from build123d import *
from build123d.topology import SkipClean

# Parameters (mm, degrees)
SKETCH1_W               = 29.21
SKETCH1_H               = 55.1434
BOSS_EXTRUDE1_DEPTH     = 55.88
SKETCH2_R               = 12.065
CUT_REVOLVE1_ANGLE      = 90
SKETCH3_R               = 25.4
CUT_EXTRUDE1_DEPTH      = 43.18
CUT_EXTRUDE4_DEPTH      = 2.0955
CUT_EXTRUDE4_DEPTH_BACK = 0.508
SKETCH6_R               = 23.8125
SKETCH7_R               = 2.6543
CUT_EXTRUDE5_DEPTH      = 7.62
CHAMFER1_SIZE           = 7.62
CHAMFER1_SIZE2          = 13.198227154
SKETCH8_R               = 2.6543
CUT_EXTRUDE6_DEPTH      = 7.62
SKETCH9_R               = 2.6543
CUT_EXTRUDE7_DEPTH      = 7.62


with BuildPart() as part:
    # Sketch1 → Boss-Extrude1 (new body)
    with BuildSketch(Plane(origin=(0, 0, 0), x_dir=(1, 0, 0), z_dir=(0, 1, 0))):
        with Locations((0, -27.5717)):
            Rectangle(SKETCH1_W, SKETCH1_H)
    extrude(amount=BOSS_EXTRUDE1_DEPTH)

    # Sketch2 → Cut-Revolve1 (revolve, cut)
    with BuildSketch(Plane(origin=(0, 0, 0), x_dir=(-1, 0, 0), z_dir=(0, 0, -1))):
        with Locations((0, 40.5384)):
            Circle(SKETCH2_R)
    revolve(axis=Axis((14.605, 0, 0), (1, 0, 0)), revolution_arc=CUT_REVOLVE1_ANGLE, mode=Mode.SUBTRACT)

    # Sketch3 → Cut-Extrude1 (cut)
    with BuildSketch(Plane(origin=(0, 55.88, 0), x_dir=(1, 0, 0), z_dir=(0, 1, 0))):
        with Locations((-29.0576, 0)):
            Circle(SKETCH3_R)
        with Locations((29.0576, 0)):
            Circle(SKETCH3_R)
    extrude(amount=-CUT_EXTRUDE1_DEPTH, mode=Mode.SUBTRACT)

    # Sketch6 → Cut-Extrude4 (cut, two sides: drawn at the far end of the back side and taken through both)
    with SkipClean():  # the faces are left unmerged after this step: merging them gives an invalid solid
        with BuildSketch(Plane(origin=(0, 8.4328, 0), x_dir=(-1, 0, 0), z_dir=(0, -1, 0)).offset(-CUT_EXTRUDE4_DEPTH_BACK)):
            with Locations((0, -60.8584)):
                Circle(SKETCH6_R)
        extrude(amount=CUT_EXTRUDE4_DEPTH + CUT_EXTRUDE4_DEPTH_BACK, mode=Mode.SUBTRACT)

    # Sketch7 → Cut-Extrude5 (cut)
    with SkipClean():  # the faces are left unmerged after this step: merging them gives an invalid solid
        with BuildSketch(Plane.XZ):
            with Locations(Location((0, 6.35, 0), (0, 0, 270))):
                Circle(SKETCH7_R)
            with Locations(Location((-8.128, 21.59, 0), (0, 0, 270))):
                Circle(SKETCH7_R)
            with Locations(Location((8.128, 21.59, 0), (0, 0, 270))):
                Circle(SKETCH7_R)
        extrude(amount=-CUT_EXTRUDE5_DEPTH, mode=Mode.SUBTRACT)

    # Chamfer1
    chamfer1_edges = [part.edges().sort_by_distance(p)[0] for p in [
        (-14.605, 6.35, 0),
        (14.605, 6.35, 0),
    ]]
    chamfer1_side = [part.faces().sort_by_distance(p)[0] for p in [
        (0, 9.780788916, 0),
    ]]
    chamfer(chamfer1_edges, length=CHAMFER1_SIZE, length2=CHAMFER1_SIZE2, reference=chamfer1_side[0])

    # Sketch8 → Cut-Extrude6 (cut)
    with SkipClean():  # the faces are left unmerged after this step: merging them gives an invalid solid
        with BuildSketch(Plane(origin=(0, 55.88, 0), x_dir=(1, 0, 0), z_dir=(0, 1, 0))):
            with Locations(Location((-7.62, -48.2854, 0), (0, 0, 270))):
                Circle(SKETCH8_R)
            with Locations(Location((7.62, -48.2854, 0), (0, 0, 270))):
                Circle(SKETCH8_R)
        extrude(amount=-CUT_EXTRUDE6_DEPTH, mode=Mode.SUBTRACT)

    # Sketch9 → Cut-Extrude7 (cut)
    with SkipClean():  # the faces are left unmerged after this step: merging them gives an invalid solid
        with BuildSketch(Plane.ZY.offset(14.605)):
            with Locations((47.5234, 43.18)):
                Circle(SKETCH9_R)
            with Locations((47.5234, 30.48)):
                Circle(SKETCH9_R)
        extrude(amount=-CUT_EXTRUDE7_DEPTH, mode=Mode.SUBTRACT)


solid = part.part
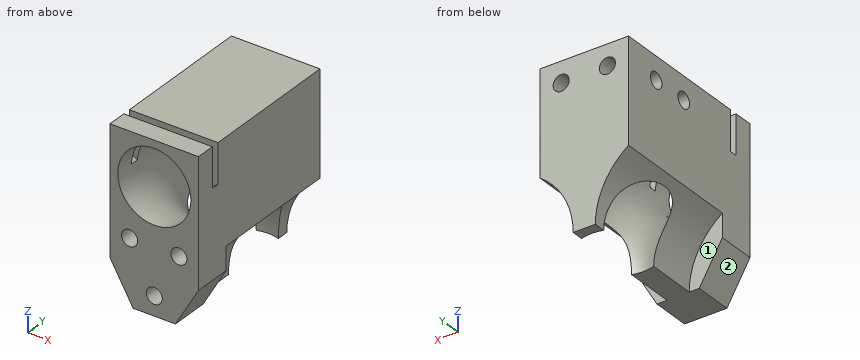
Build history of the part. All positions in model axes, mm. Face numbers are marked on the shaded views. A direction names the side the tool comes from. Give positions to 0.01 mm unless a question says otherwise; leave off trailing zeros. Loops run counter-clockwise (first coordinate to the right, second up) from the corner with the lowest first, then second, coordinate; pieces in that order, holes last. Notation, with made-up numbers: (1.25, -28) - (39.25, -28) arc R24 ccw to (39.25, -3) - close; hole circle Ø7 at (-19, 45). An arc over 180 degrees is marked (long way). Write item = value, one per line. Start each with the question number.
1) Probe probe 1 along Y at (x, z) = (-12.25, 44); probe 2 along Y at (x, z) = (-9.5, 21); probe 3 along X at (y, z) = (52, 47) (3 decimals). List the from-to ranges inside material, lowest first. Write a range as from..to.
2) Tool access for the marked faces 1 and 2: list every direction of +Z, -Z, +X, -X, +Y, -Y with a clear straight run to the whole face (end or side of a thin tool).
3) Band-saw the part on A-A on x = 0. Give the cut face in (y, z).
4) Drop flat-ended pins along their axis: pin 1 Ø1 at (x, y) = (-11, 24.5) entering from -Z; pin 2 Ø16.5 at (x, z) = (-6, 45.5) entering from -Y; pin 3 Ø4 at (x, z) = (7.62, 48.29) entering from +Y; pin 4 Ø4 at (x, z) = (-0.5, 6) entering from -Y. Give the stop position or say it passes through.
5) Band-saw the part on B-B on z = 44. Count the separate pieces of the cut face and the enclosed holes in it, plus the area to 3 significant figures.
Final values:
q1.probe_1 = 0..6.34, 8.94..55.88
q1.probe_2 = 7.62..25.59, 43.14..55.88
q1.probe_3 = -14.605..-9.942, -5.298..5.298, 9.942..14.605
q2.face_1 = -Z, -X, +Y
q2.face_2 = -Z, -X, +Y, -Y
q3.outline = (0, 0) - (28.47, 0) arc R28.47 ccw to (0, 28.47) - (0, 9) - (7.62, 9) - (7.62, 3.7) - (0, 3.7) - close; (0, 52.6) arc R52.6 cw to (6.34, 52.22) - (6.34, 55.14) - (0, 55.14) - close; (8.94, 51.84) arc R52.6 cw to (52.6, 0) - (55.88, 0) - (55.88, 55.14) - (8.94, 55.14) - close
q4.pin_1 = 17.34
q4.pin_2 = 0
q4.pin_3 = 48.26
q4.pin_4 = 7.62
q5.separate_pieces = 3
q5.enclosed_holes = 0
q5.area = 1,060 mm²
